Geometry: final body of the model. Coordinates: model frame, mm. Face numbers are marked on the shaded views. A direction names the side the tool comes from. Coordinates: 2 decimals unless noted, no trailing zeros. Order: outer loops, then holes, each group sorted by start corner. A loop starts at its lowest first (then second) coordinate and runs counter-clockwise, first axis right, second up. Notation, with made-up numbers: (80.25, 39.5) -> (95.25, 39.5) arc R4 ccw to (95.25, 45.5) -> close; hole circle Ø4 at (-10, -16.5). An arc over 180 degrees is marked (long way). Use one line per item in the form item = value.
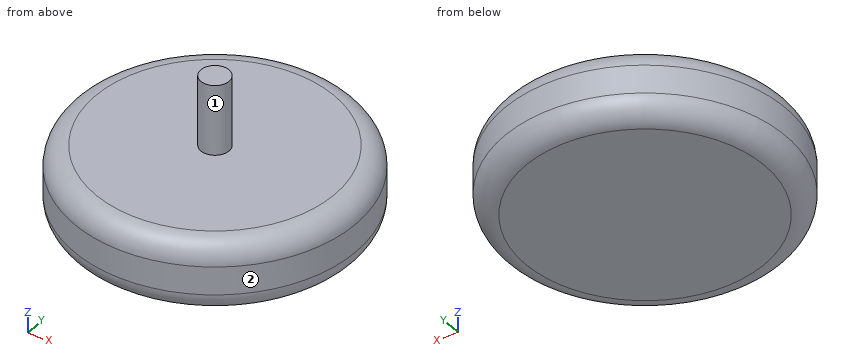
```python
from build123d import *

# Parameters (mm, degrees)
SKETCH_1_R      = 100
EXTRUDE_1_DEPTH = 50
SKETCH_2_R      = 10
EXTRUDE_2_DEPTH = 50
FILLET_1_R      = 15


with BuildPart() as part:
    # 草图1 → 凸台-拉伸1 (new body)
    with BuildSketch(Plane.XY):
        Circle(SKETCH_1_R)
    extrude(amount=EXTRUDE_1_DEPTH)

    # 草图2 → 凸台-拉伸2 (add)
    with BuildSketch(Plane.XY.offset(50)):
        Circle(SKETCH_2_R)
    extrude(amount=EXTRUDE_2_DEPTH)

    # 圆角1
    fillet_1_edges = [part.edges().sort_by_distance(p)[0] for p in [
        (-100, 0, 0),
        (-100, 0, 50),
    ]]
    fillet(fillet_1_edges, radius=FILLET_1_R)


solid = part.part
```
1) Material intervals for probe 1 along Z at (x, y) = (51, 53.5); probe 2 along Y at (x, z) = (13.5, 5); probe 3 along X at (y, z) = (4.5, 78), sorted ascending. Write a range as from..to.
Results found:
probe_1 = 0..50
probe_2 = -95.23..95.23
probe_3 = -8.93..8.93
2) Contact query for flat-ended pins moving along their axis: P1, Ø1, axis at x = -39.5, z = 37.5, coming from the -Y side; P2, Ø3, axis at x = 7.5, y = 80, coming from the +Z side; P3, Ø2, axis at y = -51.5, z = 39, coming from the -X side. Output: stop coordinate, or through.
Results found:
P1 = -91.87
P2 = 50
P3 = -85.75
3) Section C-C, the plane z = 72. Output: boundary loops of the cut face in (x, y), and give its area (3 significant figures).
Results found:
outline = circle Ø20 at (0, 0)
area = 314 mm2
4) Section D-D, the plane z = 44. Output: boundary loops of the cut face in (x, y), and give its area (3 significant figures).
Results found:
outline = circle Ø194 at (0, 0)
area = 29,600 mm2
5) Access query for the marked faces 1 and 2. Directions: +Z, -Z, +X, -X, +Y, -Y. A direction counts if a zero-diameter tool reaches every point of the face in a straight line with its end or side. Return the directions, or none.
Results found:
face_1 = +Z
face_2 = +Z, -Z
6) Section A-A, the plane x = 0. Output: boundary loops of the cut face in (y, z).
Results found:
outline = (-100, 15) arc R15 ccw to (-85, 0) -> (85, 0) arc R15 ccw to (100, 15) -> (100, 35) arc R15 ccw to (85, 50) -> (10, 50) -> (10, 100) -> (-10, 100) -> (-10, 50) -> (-85, 50) arc R15 ccw to (-100, 35) -> close
